Answer from the drawing. Dimensions are ordinates in mm from the lowest x, y and z of the part. Coordinates: 2 decimals unless noted, no trailing zeros. Order: outer loops, then holes, each group sorted by start corner. A loop starts at its lowest first (then second) coordinate and runs counter-clockwise, first axis right, second up. Notation, with made-up numbers: (-29, 57) -> (-10, 57) arc R19 cw to (-10, 70) -> close; hole circle Ø1 at (-27.75, 63.5). An arc over 180 degrees is marked (long way). Answer in a Markdown table with one row per item.
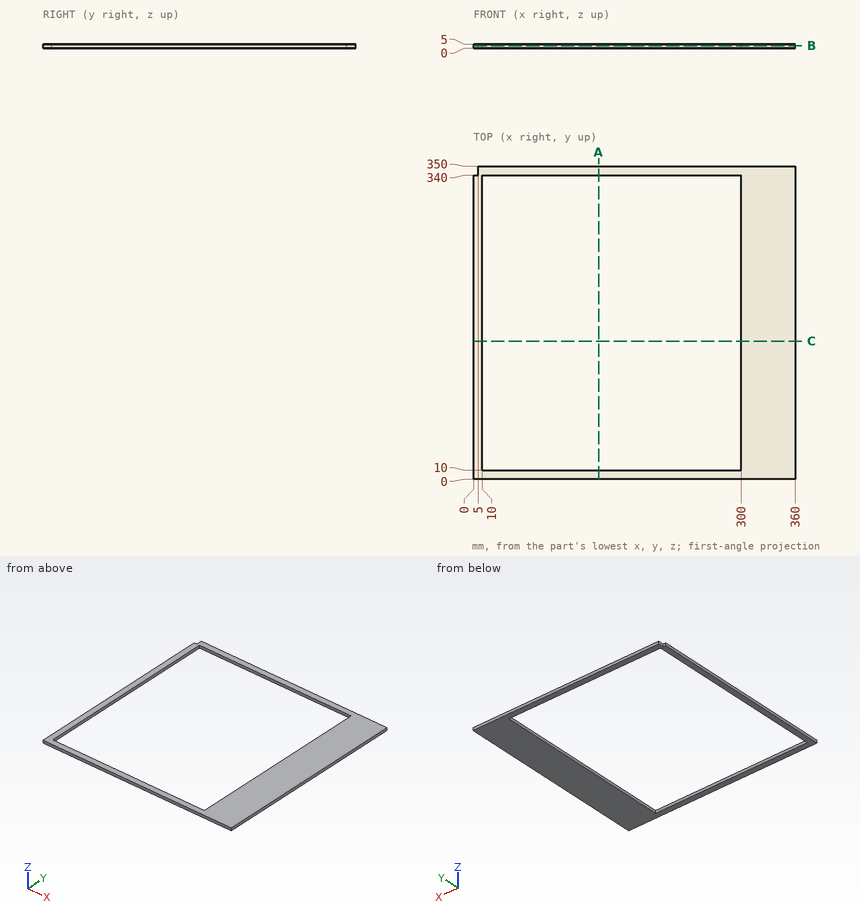
Q1. The part is cut by section A-A (x = 140). Write down the section's boundary in (y, z), then the cut area to 3 significant figures.
Outcome:
| item | result |
|---|---|
| outline | (0, 0) -> (10, 0) -> (10, 5) -> (0, 5) -> close; (340, 0) -> (350, 0) -> (350, 5) -> (340, 5) -> close |
| area | 100 mm² |
Q2. The part is cut by section B-B (z = 3.15). Write down the section's boundary in (x, y).
Outcome:
| item | result |
|---|---|
| outline | (0, 0) -> (360, 0) -> (360, 350) -> (5, 350) -> (5, 340) -> (0, 340) -> close; hole (10, 10) -> (300, 10) -> (300, 340) -> (10, 340) -> close |
Q3. Consider line 1 (X direction, y = 103.5, z = 2.9); line 2 (Y direction, x = 54, z = 2.3). Determine where each line is inside the solid, lowest interval first.
Outcome:
| item | result |
|---|---|
| line 1 | 0 to 10, 300 to 360 |
| line 2 | 0 to 10, 340 to 350 |
Q4. Given pin 1 (2.5 mm diameter, centred on x = 2.5, z = 3.5, fed in from +Y), flat-ended and moving along its own axis, determine where the tip first touches the part or whether it passes through.
Outcome:
| item | result |
|---|---|
| pin 1 | y = 340 |
Q5. The part is cut by section C-C (y = 154.5). Write down the section's boundary in (x, z).
Outcome:
| item | result |
|---|---|
| outline | (0, 0) -> (10, 0) -> (10, 5) -> (0, 5) -> close; (300, 0) -> (360, 0) -> (360, 5) -> (300, 5) -> close |
